Verification items for the finished model (mm, model axes). A direction names the side the tool comes from. Round coordinates to 2 decimals unless told otherwise and drop trailing zeros. Write each loop counter-clockwise with the first axis right and the second up, starting at its lowest first coordinate (ties: lowest second). Pieces come first, ordered by that corner, then holes. Notation, with made-up numbers: M -13,68.5 L 4,68.5 A9 cw 4,74.5 Z; hole C 17.5,-14 d1. An arc over 180 degrees is marked long. Answer in a Markdown table with one row per item. Add a question column.
1. Sectioned sample at C-C on y = 14.5. Record the cut outline in (x, z).
2. Go/stop test with flat-tipped pins: pin 1 Ø8 at (x, y) = (28, 1) entering from +Z; pin 2 Ø1.2 at (x, z) = (16, 1) entering from -Y; pin 3 Ø1.7 at (y, z) = (17.5, 1) entering from -X. Record where each tip stops, or that it passes through.
3. Set-up check for faces 5 (the flat face through (-3.429, 16, -1)), 6 (the flat face through (21.183, 16, 1)): record each of +Z, -Z, +X, -X, +Y, -Y from which the full face is reachable in a straight line by a thin tool's end or side.
4. Material ranges on probe 1 along Y at (x, z) = (0, -1.9); probe 2 along X at (y, z) = (0.5, -1.3); probe 3 along Y at (x, z) = (34, -0.1), recorded low to high.
5. Sectioned sample at D-D on x = 18. Record the cut outline in (y, z), plus the area to 3 significant figures.
6. Draft check along Y on faces 1 (the flat face through (11.583, 16, 1)), 2 (the flat face through (16, 21.056, 1)), 3 (the flat face through (16, 11.456, 1)), 4 (the cylindrical face through (31.865, 32.541, -1.288)). Enter one of: pulls with the +Y half, pulls with the -Y half, needs draft (parallel to the pull), parting line crosses it, or undercut.
7. Sectioned sample at A-A on x = 0. Record the cut outline in (y, z), plus the area to 3 significant figures.
```python
from build123d import *

# Parameters (mm, degrees)
SCHIZZO2_W                   = 39.87805
SCHIZZO2_H                   = 39.87805
ESTRUSIONE_ESTRUSIONE1_DEPTH = 2.54
FORO_FILETTATO_M3X0_5_1_D    = 2.5
SCHIZZO5_W                   = 9.6
SCHIZZO5_H                   = 9.6
ESTRUSIONE_ESTRUSIONE2_DEPTH = 1.54


with BuildPart() as part:
    # Schizzo2 → Estrusione-Estrusione1 (new body)
    with BuildSketch(Plane.XY):
        with Locations((16.509975, 16.509975)):
            Rectangle(SCHIZZO2_W, SCHIZZO2_H)
    extrude(amount=-ESTRUSIONE_ESTRUSIONE1_DEPTH)

    # Foro filettato M3x0.5-1 (through all)
    with Locations(Plane.XY):
        with Locations((0, 33.02), (33.02, 33.02), (33.02, 0), (0, 0)):
            Hole(FORO_FILETTATO_M3X0_5_1_D / 2)

    # Schizzo5 → Estrusione-Estrusione2 (add)
    with BuildSketch(Plane.XY):
        with Locations((16.383, 16.256)):
            Rectangle(SCHIZZO5_W, SCHIZZO5_H)
    extrude(amount=ESTRUSIONE_ESTRUSIONE2_DEPTH)


solid = part.part
```
Geometry check:
| question | item | result |
|---|---|---|
| 1 | outline | M -3.43,-2.54 L 36.45,-2.54 L 36.45,0 L 21.18,0 L 21.18,1.54 L 11.58,1.54 L 11.58,0 L -3.43,0 Z |
| 2 | pin 1 | stops at z = 0 |
| 2 | pin 2 | stops at y = 11.46 |
| 2 | pin 3 | stops at x = 11.58 |
| 3 | face 5 | +Z, -Z, -X, +Y, -Y |
| 3 | face 6 | +Z, +X, +Y, -Y |
| 4 | probe 1 | y = -3.43 to -1.25, 1.25 to 31.77, 34.27 to 36.45 |
| 4 | probe 2 | x = -3.43 to -1.15, 1.15 to 31.87, 34.17 to 36.45 |
| 4 | probe 3 | y = -3.43 to -0.78, 0.78 to 32.24, 33.8 to 36.45 |
| 5 | outline | M -3.43,-2.54 L 36.45,-2.54 L 36.45,0 L 21.06,0 L 21.06,1.54 L 11.46,1.54 L 11.46,0 L -3.43,0 Z |
| 5 | area | 116 mm2 |
| 6 | face 1 | needs draft |
| 6 | face 2 | pulls with the +Y half |
| 6 | face 3 | pulls with the -Y half |
| 6 | face 4 | undercut |
| 7 | outline | M -3.43,-2.54 L -1.25,-2.54 L -1.25,0 L -3.43,0 Z; M 1.25,-2.54 L 31.77,-2.54 L 31.77,0 L 1.25,0 Z; M 34.27,-2.54 L 36.45,-2.54 L 36.45,0 L 34.27,0 Z |
| 7 | area | 88.6 mm2 |
